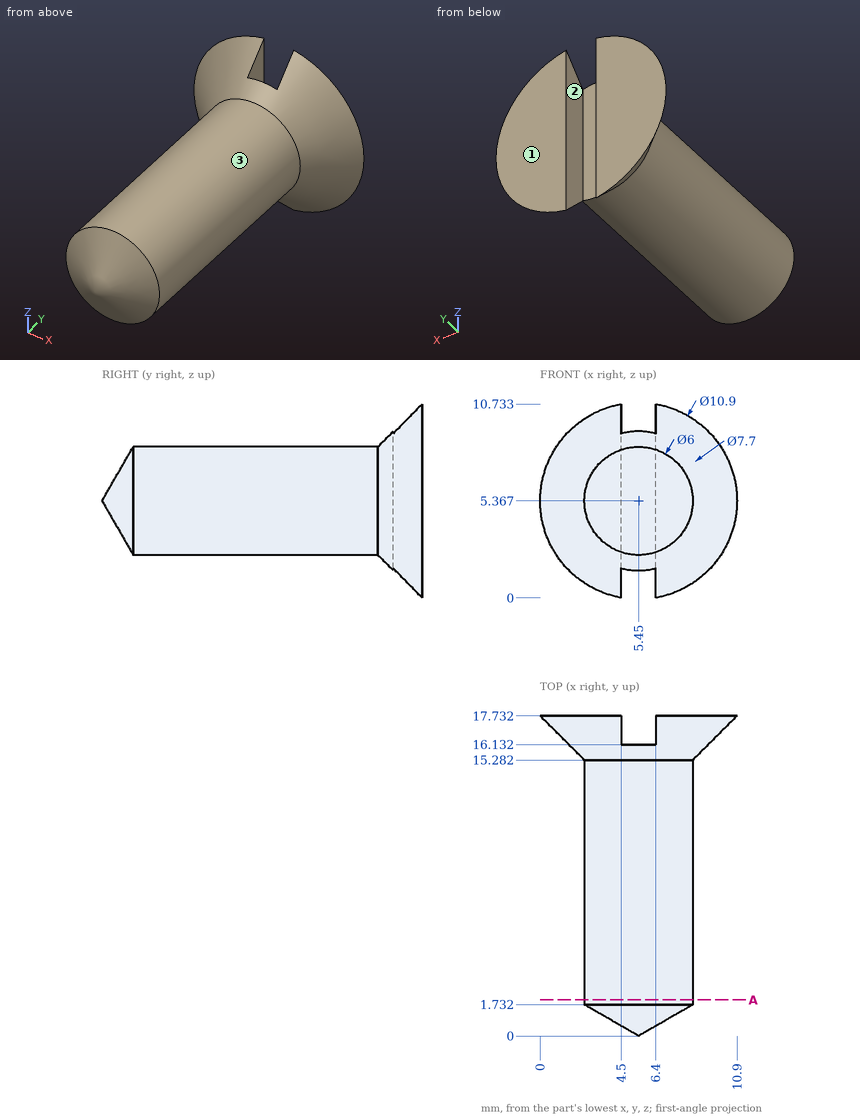
Check sheet for the drawn part. Datum: minimum x, y, z corner. Units: mm. Round coordinates to 2 decimals unless told otherwise and drop trailing zeros. Loops run counter-clockwise (first coordinate to the right, second up) from the corner with the lowest first, then second, coordinate; pieces in that order, holes last. Notation, with made-up numbers: (84.25, 34.25) - (136.25, 34.25) arc R22 cw to (136.25, 41.25) - close; hole circle Ø8 at (48, -10). An arc over 180 degrees is marked (long way). Answer as a JSON object with one key per item and string values. Group by question number.
Q1. Sectioned sample at A-A, the plane y = 2. Enter the section's corners in (x, z), plus the area to 3 significant figures.
Q2. Scan lines: line 1 along X through (y, z) = (14.5, 5.25); line 2 along X through (y, z) = (11.25, 4.25) (1 decimal); line 3 along Y through (x, z) = (3.75, 8) (1 decimal). Record each from-to range of solid material in increasing order. Write a range as [from, to].
Q3. Mould release check, pull along X, two halves, no side actions. Record for the marked faces 1, 2 and 3: released by +X, released by -X, zero draft, split by the parting line, or undercut.
Q4. Gauge pin test, flat ends, axial feed: P1, Ø0.8, axis at y = 16.5, z = 4.5, coming from the -X side; P2, Ø0.8, axis at y = 16.5, z = 5.5, coming from the +X side (1 decimal); P3, Ø2, axis at x = 9, z = 4.5, coming from the -Y side. Record the tip position at first contact, or that the pin passes through.
Solution:
{
 "1": {"outline": "circle Ø6 at (5.45, 5.37)", "area": "28.3 mm²"},
 "2": {"line 1": "x = [2.45, 8.45]", "line 2": "x = [2.7, 8.2]", "line 3": "y = [15.4, 17.7]"},
 "3": {"face 1": "zero draft", "face 2": "undercut", "face 3": "split by the parting line"},
 "4": {"P1": "stops at x = 0.91", "P2": "stops at x = 10.1", "P3": "stops at y = 1.53"}
}
